Design review of the part built by this model. Coordinates are the model's own, in mm. Face numbers are marked on the shaded views. A direction names the side the tool comes from. Give positions to 0.01 mm unless a question says otherwise; leave off trailing zeros. Loops run counter-clockwise (first coordinate to the right, second up) from the corner with the lowest first, then second, coordinate; pieces in that order, holes last.
Autodesk Inventor part; units mm, degrees
ref_plane "YZ Plane" through (0, 0, 0) normal (1, 0, 0) x (0, 1, 0)
ref_plane "XZ Plane" through (0, 0, 0) normal (0, 1, 0) x (-1, 0, 0)
ref_plane "XY Plane" through (0, 0, 0) normal (0, 0, 1) x (1, 0, 0)
sketch "Sketch1" plane through (0, 0, 0) normal (0, 0, 1) x (1, 0, 0)
  line L0 (0, 0) -> (80.4347, 67.4927)
  line L1 (80.4347, 67.4927) -> (160.8693, 0)
  line L2 (0, 0) -> (279.217, 0) construction
  line L3 (160.8693, 0) -> (162.1549, 1.5321)
  line L4 (162.1549, 1.5321) -> (80.4347, 70.1035)
  line L5 (-1.2856, 1.5321) -> (80.4347, 70.1035)
  line L6 (0, 0) -> (-1.2856, 1.5321)
  dimension "d0" = 105
  dimension "d1" = 105
  dimension "d2" = 100
  dimension "d3" = 2
  dimension "d4" = 90
  dimension "d7" = 2
  dimension "d8" = 90
extrude "Extrusion1" add sketch "Sketch1" against normal blind 300
properties part number "techo" material "PET Plastic"
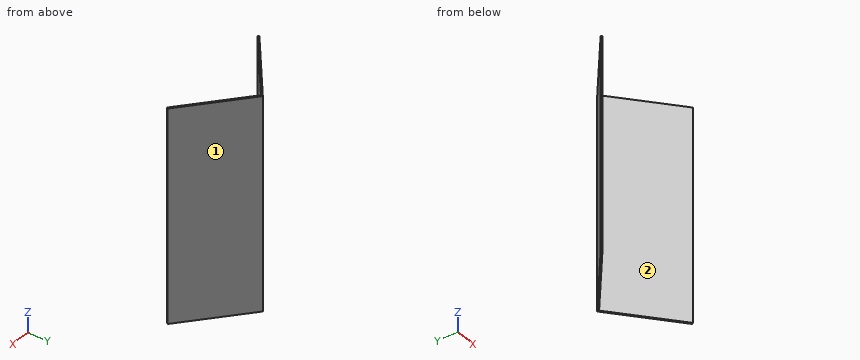
Q1. Take a section at A-A (y = 17). Give the boundary of the cut face in (x, z).
Results:
outline: (17.15, -300) - (20.26, -300) - (20.26, 0) - (17.15, 0) - close; (140.61, -300) - (143.72, -300) - (143.72, 0) - (140.61, 0) - close
Q2. Take a section at C-C (y = 46). Give the boundary of the cut face in (x, z).
Results:
outline: (51.71, -300) - (54.82, -300) - (54.82, 0) - (51.71, 0) - close; (106.05, -300) - (109.16, -300) - (109.16, 0) - (106.05, 0) - close
Q3. Tool access review of the marked faces 1 and 2: name each direction out of +Z, -Z, +X, -X, +Y, -Y from which nothing blocks a thin tool from reaching the whole face with its end or side.
Results:
face 1: +Z, -Z, +X, +Y
face 2: +Z, -Z, -Y
Q4. Take a section at B-B (z = -32). Give the boundary of the cut face in (x, y).
Results:
outline: (-1.29, 1.53) - (0, 0) - (80.43, 67.49) - (160.87, 0) - (162.15, 1.53) - (80.43, 70.1) - close
Q5. Insertion check: pin 1 (8 mm diameter, centred on y = 21.5, z = -259, fed in from -X); pin 2 (2 mm diameter, centred on y = 59, z = -84.5, fed in from +X); pin 3 (10 mm diameter, centred on x = 105, z = -89, fed in from +Y). Each pin has a flat end and moves straight along its axis. Give the tip position at first contact, or say it passes through.
Results:
pin 1: stops at x = 17.74
pin 2: stops at x = 94.86
pin 3: stops at y = 53.69
Q6. Wall thickness on line 1 (X direction, y = 37, z = -168.5); line 2 (X direction, y = 14.5, z = -114.5); line 3 (Y direction, x = 16, z = -252): over which ranges is each line inside the solid? List them lowest first.
Results:
line 1: x = 40.98 to 44.09, 116.77 to 119.89
line 2: x = 14.17 to 17.28, 143.59 to 146.7
line 3: y = 13.43 to 16.04
Q7. Take a section at D-D (x = 32.5). Give the boundary of the cut face in (y, z).
Results:
outline: (27.27, -300) - (29.88, -300) - (29.88, 0) - (27.27, 0) - close
